Geometry check sheet. Reference: the model listing, model coordinates, mm. Face numbers are marked on the shaded views. A direction names the side the tool comes from. Give positions to 0.01 mm unless a question says otherwise; leave off trailing zeros. Write each loop counter-clockwise with the first axis right and the second up, starting at its lowest first coordinate (ties: lowest second). Pieces come first, ordered by that corner, then holes. Notation, with made-up numbers: M 45.25,69 L 83.25,69 A8 cw 83.25,74 Z; hole C -11.5,-20 d7. An arc over 180 degrees is marked long. One line per item, written item: value. Start each with the question number.
1. Scan lines: line 1 (X direction, y = 0, z = -4); line 2 (Y direction, x = -19, z = 1.5); line 3 (Z direction, x = 38, y = -0.5). Record each from-to range of solid material in increasing order.
2. Tool access check on the marked faces 1 and 2. Record the directions out of +Z, -Z, +X, -X, +Y, -Y that give a thin tool (end or side, any length) a straight path to the whole face; none if there is none.
3. Cross-section at B-B on z = 0. Record the cut outline in (x, y).
4. Gauge pin test, flat ends, axial feed: pin 1 (6 mm diameter, centred on x = -4.5, z = 11, fed in from +Y); pin 2 (1.5 mm diameter, centred on x = -15.5, y = 12, fed in from -Z); pin 3 (1 mm diameter, centred on x = -5, y = -8, fed in from +Z). Record the tip position at first contact, or that the pin passes through.
5. Cross-section at A-A on y = 0. Record the cut outline in (x, z), then the cut area to 3 significant figures.
6. Cross-section at D-D on x = -22.5. Record the cut outline in (y, z), then the cut area to 3 significant figures.
7. Cross-section at C-C on x = 40.5. Record the cut outline in (y, z).
8. Release check for a two-part mould opening along X. For the marked faces 3, 4 and 5 record: pulls with the +X half, pulls with the -X half, needs draft (parallel to the pull), parting line crosses it, or undercut.
from build123d import *

# Parameters (mm, degrees)
SCHIZZO1_R             = 20
ESTRUSIONE1_DEPTH      = 52
SCHIZZO2_R             = 18
ESTRUSIONE2_DEPTH      = 32
ESTRUSIONE5_DEPTH      = 60.194594348
ESTRUSIONE5_DEPTH_BACK = 60.194594348
SCHIZZO5_R             = 4
SMUSSO2_SIZE           = 2
SCHIZZO3_R             = 17
ESTRUSIONE3_DEPTH      = 2
SCHIZZO4_R             = 18
ESTRUSIONE4_DEPTH      = 4
SMUSSO1_SIZE           = 2
SCHIZZO6_R             = 24.071831276
ESTRUSIONE6_DEPTH      = 10


with BuildPart() as part:
    # Schizzo1 → Estrusione1 (new body)
    with BuildSketch(Plane(origin=(0, 0, 0), x_dir=(0, 0, -1), z_dir=(1, 0, 0))):
        with Locations(Location((0, 0, 0), (0, 0, 180))):
            Circle(SCHIZZO1_R)
    extrude(amount=ESTRUSIONE1_DEPTH)

    # Schizzo2 → Estrusione2 (add)
    with BuildSketch(Plane.ZY):
        with Locations(Location((0, 0, 0), (0, 0, 180))):
            Circle(SCHIZZO2_R)
    extrude(amount=ESTRUSIONE2_DEPTH)

    # Schizzo5 → Estrusione5 (cut, two sides: drawn at the far end of the back side and taken through both)
    with BuildSketch(Plane.XY.offset(-ESTRUSIONE5_DEPTH_BACK)):
        with Locations((-22.5, 0)):
            Circle(SCHIZZO5_R)
    extrude(amount=ESTRUSIONE5_DEPTH + ESTRUSIONE5_DEPTH_BACK, mode=Mode.SUBTRACT)

    # Smusso2
    smusso2_edges = [part.edges().sort_by_distance(p)[0] for p in [
        (-32, 0, 18),
    ]]
    chamfer(smusso2_edges, length=SMUSSO2_SIZE)

    # Schizzo3 → Estrusione3 (add)
    with BuildSketch(Plane.ZY.offset(32)):
        Circle(SCHIZZO3_R)
    extrude(amount=ESTRUSIONE3_DEPTH)

    # Schizzo4 → Estrusione4 (add)
    with BuildSketch(Plane.ZY.offset(34)):
        with Locations(Location((0, 0, 0), (0, 0, 180))):
            Circle(SCHIZZO4_R)
    extrude(amount=ESTRUSIONE4_DEPTH)

    # Smusso1
    smusso1_edges = [part.edges().sort_by_distance(p)[0] for p in [
        (-38, 0, 18),
    ]]
    chamfer(smusso1_edges, length=SMUSSO1_SIZE)

    # Schizzo6 → Estrusione6 (cut)
    with BuildSketch(Plane(origin=(-32, 0, 0), x_dir=(0, 0, -1), z_dir=(1, 0, 0))):
        Circle(SCHIZZO6_R)
    extrude(amount=-ESTRUSIONE6_DEPTH, mode=Mode.SUBTRACT)


solid = part.part
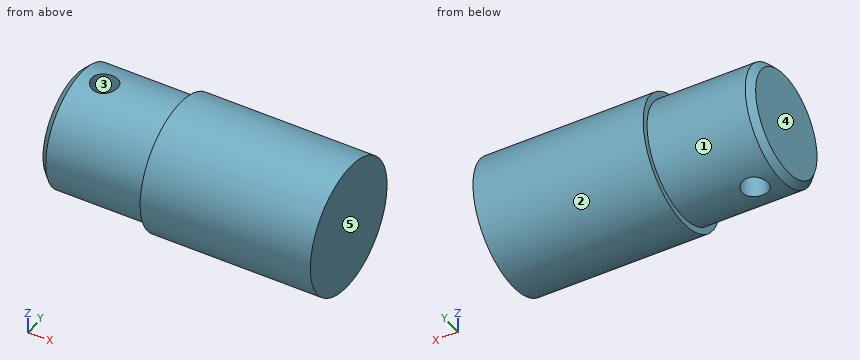
Report:
1. line 1: x = -32 to -26.5, -18.5 to 52
1. line 2: y = -17.94 to -1.94, 1.94 to 17.94
1. line 3: z = -19.99 to 19.99
2. face 1: -X
2. face 2: +X, -X
3. outline: M -32,-16 L -30,-18 L 0,-18 L 0,-20 L 52,-20 L 52,20 L 0,20 L 0,18 L -30,18 L -32,16 Z; hole C -22.5,0 d8
4. pin 1: stops at y = 16.12
4. pin 2: stops at z = -14.05
4. pin 3: stops at z = 16.36
5. outline: M -32,-16 L -30,-18 L -26.5,-18 L -26.5,18 L -30,18 L -32,16 Z; M -18.5,-18 L 0,-18 L 0,-20 L 52,-20 L 52,20 L 0,20 L 0,18 L -18.5,18 Z
5. area: 2,940 mm^2
6. outline: M -4,-17.55 L -4,17.55 A18 ccw Z; M 4,-17.55 A18 ccw 4,17.55 Z
6. area: 732 mm^2
7. outline: C 0,0 d40
8. face 3: undercut
8. face 4: pulls with the -X half
8. face 5: pulls with the +X half
